from build123d import *


with BuildPart() as part:
    # Sketch2 → Revolve2 (revolve)
    with BuildSketch(Plane.XY, mode=Mode.PRIVATE) as revolve2_sk:
        with BuildLine():
            Line((0, 1.2), (50, 4.696340597))
            Line((50, 4.696340597), (50, 6.696340597))
            Line((50, 6.696340597), (1.851094968, 3.32944117))
            ThreePointArc((1.851094968, 3.32944117), (0.484525778, 2.648094905), (0, 1.2))
        make_face()
    revolve(revolve2_sk.sketch.rotate(Axis((-19.275847123, 0, 0), (1, 0, 0)), 90), axis=Axis((-19.275847123, 0, 0), (1, 0, 0)))

    # Sketch3 → Revolve3 (revolve)
    with BuildSketch(Plane.XY, mode=Mode.PRIVATE) as revolve3_sk:
        Polygon((50, 4.695121509), (180, 9.234821543), (180, 11.236040631), (50, 6.696340597), align=None)
    revolve(revolve3_sk.sketch.rotate(Axis((50, 0, 0), (-1, 0, 0)), 90), axis=Axis((50, 0, 0), (-1, 0, 0)))

    # SurfaceCut3
    split(bisect_by=Plane(origin=(50, 0, 0), x_dir=(0, 0, -1), z_dir=(1, 0, 0)), keep=Keep.TOP)

    # Sketch4 → Revolve4 (revolve)
    with BuildSketch(Plane.XY, mode=Mode.PRIVATE) as revolve4_sk:
        Polygon((50, 6.195119648), (47, 5.484118263), (50, 5.196340597), align=None)
    revolve(revolve4_sk.sketch.rotate(Axis((50, 0, 0), (-1, 0, 0)), 90), axis=Axis((50, 0, 0), (-1, 0, 0)))


solid = part.part
Geometry: final body of the model. Coordinates: model frame, mm. A direction names the side the tool comes from. Give positions to 0.01 mm unless a question says otherwise; leave off trailing zeros. Write each loop counter-clockwise with the first axis right and the second up, starting at its lowest first coordinate (ties: lowest second). Pieces come first, ordered by that corner, then holes.
(1) Cut plane C-C, the plane x = 103. Return loops of the section in (y, z), then the cut area to 3 significant figures.
(2) Ray query, line 1 (Y direction, x = 165.5, z = 7.5) (3 decimals); line 2 (Z direction, x = 124.5, y = 5.5) (3 decimals); line 3 (Y direction, x = 119.5, z = 3.75). Return the intervals inside material, ascending.
(3) Access query for faces 1 (the flat face through (180, -4.2, -8.4)), 2 (the flat face through (50, 3, 4)), 3 (the conical face through (115.91, 6.83, 1.52)). Directions: +Z, -Z, +X, -X, +Y, -Y. A direction counts if a zero-diameter tool reaches every point of the face in a straight line with its end or side. Return the directions, or none.
(4) Cut plane A-A, the plane y = 0. Return loops of the section in (x, z), then the cut area to 3 significant figures.
(5) First-contact query: P1, Ø6, axis at x = 82, y = -1.5, coming from the -Z side; P2, Ø6, axis at y = 5.5, z = -3, coming from the -X side; P3, Ø3, axis at y = 1.5, z = 1, coming from the -X side; P4, Ø12, axis at x = 96, y = 1.5, coming from the +Z side. Flat tips, straight axial feed; report the tip coordinate or a pass-through.
Values follow:
1. outline: circle Ø17.09 at (0, 0); hole circle Ø13.09 at (0, 0)
1. area: 94.9 mm2
2. line 1: y = -7.673 to -4.465, 4.465 to 7.673
2. line 2: z = -7.497 to -4.795, 4.795 to 7.497
2. line 3: y = -8.32 to -6.05, 6.05 to 8.32
3. face 1: +Z, -Z, +X, +Y, -Y
3. face 2: -X
3. face 3: +X
4. outline: (47, -5.48) - (50, -6.2) - (50, -6.7) - (180, -11.24) - (180, -9.23) - (50, -4.7) - (50, -5.2) - close; (47, 5.48) - (50, 5.2) - (50, 4.7) - (180, 9.23) - (180, 11.24) - (50, 6.7) - (50, 6.2) - close
4. area: 523 mm2
5. P1: stops at z = -7.91
5. P2: stops at x = 47
5. P3: passes through
5. P4: stops at z = 8.51
